Design review of the part built by this model. Coordinates are the model's own, in mm. Face numbers are marked on the shaded views. A direction names the side the tool comes from. Coordinates: 2 decimals unless noted, no trailing zeros. Write each loop counter-clockwise with the first axis right and the second up, starting at its lowest first coordinate (ties: lowest second). Pieces come first, ordered by that corner, then holes.
Q1. Take a section at B-B, the plane x = 0. Write out the cut boundary in (y, z), plus the area to 3 significant figures.
Q2. For pin 1 Ø1.5 at (x, y) = (-6, -3) entering from +Z; pin 2 Ø1.5 at (y, z) = (-4.5, -1) entering from -X; pin 3 Ø1 at (y, z) = (-2, 4) entering from -X, all flat-tipped, find the tip position at first contact; note any pin that passes through.
Q3. For the marked faces 1 and 2, list the 3-axis set-ups (+Z, -Z, +X, -X, +Y, -Y) from which the entire face can be reached by the end or side of a thin tool; tool diameter is ignored.
Q4. For L1, parallel to Z at x = 0, y = -4.65; L2, parallel to Y at x = 12, z = -9; L3, parallel to Z at x = 0, y = -3, list the stretches that pass through material, from the lowest coordinate up.
Q5. Take a section at A-A, the plane z = 0. Write out the cut boundary in (x, y).
Q6. Take a section at C-C, the plane y = -2.5. Write out the cut boundary in (x, z).
Q7. Take a section at D-D, the plane z = 12. Write out the cut boundary in (x, y).
from build123d import *

# Parameters (mm, degrees)
F0_R     = 11.1
F0_R_2   = 17.85
F1_DEPTH = 2
F2_DEPTH = 5
F3_R     = 4
F4_DEPTH = 1


with BuildPart() as f1:
    # F0 (on Front) → F1 (new body)
    with BuildSketch(Plane.XZ):
        Circle(F0_R)
        Circle(F0_R_2)
        Circle(F0_R, mode=Mode.SUBTRACT)
    extrude(amount=F1_DEPTH)

    # F0 (on Front) → F2 (join)
    with BuildSketch(Plane.XZ):
        Circle(F0_R)
    extrude(amount=F2_DEPTH)

    # F3 (on face) → F4 (cut)
    with BuildSketch(Plane.XZ.offset(5)):
        Circle(F3_R)
    extrude(amount=-F4_DEPTH, mode=Mode.SUBTRACT)


solid = f1.part
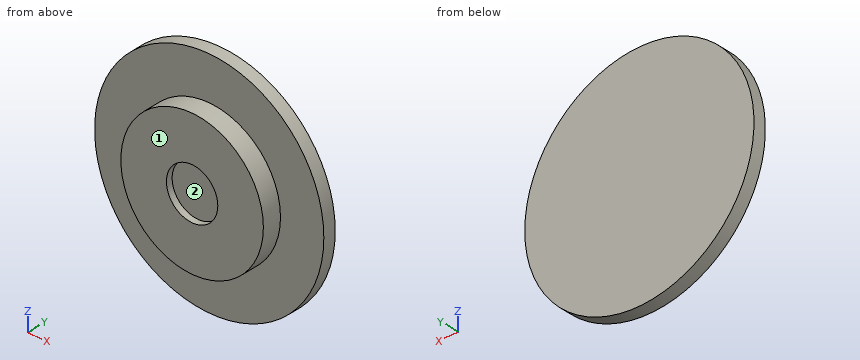
Responses:
1. outline: (-5, -11.1) - (-2, -11.1) - (-2, -17.85) - (0, -17.85) - (0, 17.85) - (-2, 17.85) - (-2, 11.1) - (-5, 11.1) - (-5, 4) - (-4, 4) - (-4, -4) - (-5, -4) - close
1. area: 130 mm2
2. pin 1: stops at z = 9.78
2. pin 2: stops at x = -11.1
2. pin 3: stops at x = -17.5
3. face 1: +Z, -Z, +X, -X, -Y
3. face 2: -Y
4. L1: z = -11.1 to -4, 4 to 11.1
4. L2: y = -2 to 0
4. L3: z = -11.1 to 11.1
5. outline: (-17.85, -2) - (-11.1, -2) - (-11.1, -5) - (-4, -5) - (-4, -4) - (4, -4) - (4, -5) - (11.1, -5) - (11.1, -2) - (17.85, -2) - (17.85, 0) - (-17.85, 0) - close
6. outline: circle Ø22.2 at (0, 0)
7. outline: (-13.21, -2) - (13.21, -2) - (13.21, 0) - (-13.21, 0) - close
